from build123d import *

# Parameters (mm, degrees)
BOX078_W               = 3
BOX078_H               = 15
BOX078_DEPTH           = 6
BOX042_W               = 3
BOX042_H               = 9
BOX042_DEPTH           = 3
BOX041_W               = 3
BOX041_H               = 15
BOX041_DEPTH           = 6
BOX044_W               = 3
BOX044_H               = 9
BOX044_DEPTH           = 3
BOX043_W               = 3
BOX043_H               = 15
BOX043_DEPTH           = 6
CUT014_PLACEMENT_ANGLE = 180
BOX040_W               = 3
BOX040_H               = 30
BOX040_DEPTH           = 15
BOX079_W               = 3
BOX079_H               = 15
BOX079_DEPTH           = 6


with BuildPart() as cube002:
    # Box078 → Box078 (new body)
    with BuildSketch(Plane(origin=(-3, 60, 15), x_dir=(1, 0, 0), z_dir=(0, 0, 1))):
        with Locations((1.5, 7.5)):
            Rectangle(BOX078_W, BOX078_H)
    extrude(amount=BOX078_DEPTH)


with BuildPart() as obj1:
    # Box042 → Box042 (new body)
    with BuildSketch(Plane(origin=(0, 3, 0), x_dir=(1, 0, 0), z_dir=(0, 0, 1))):
        with Locations((1.5, 4.5)):
            Rectangle(BOX042_W, BOX042_H)
    extrude(amount=BOX042_DEPTH)


with BuildPart() as loop004:
    # Box041 → Box041 (new body)
    with BuildSketch(Plane.XY):
        with Locations((1.5, 7.5)):
            Rectangle(BOX041_W, BOX041_H)
    extrude(amount=BOX041_DEPTH)

    # Cut013: cut obj1
    add(obj1.part, mode=Mode.SUBTRACT)


with BuildPart() as loop004_1:
    # Cut013 placement: moved
    add(loop004.part.moved(Location((30, 75, 15))))


with BuildPart() as obj2:
    # Box044 → Box044 (new body)
    with BuildSketch(Plane(origin=(0, 3, 0), x_dir=(1, 0, 0), z_dir=(0, 0, 1))):
        with Locations((1.5, 4.5)):
            Rectangle(BOX044_W, BOX044_H)
    extrude(amount=BOX044_DEPTH)


with BuildPart() as loop005:
    # Box043 → Box043 (new body)
    with BuildSketch(Plane.XY):
        with Locations((1.5, 7.5)):
            Rectangle(BOX043_W, BOX043_H)
    extrude(amount=BOX043_DEPTH)

    # Cut014: cut obj2
    add(obj2.part, mode=Mode.SUBTRACT)


with BuildPart() as loop005_1:
    # Cut014 placement: moved
    add(loop005.part.moved(Location((33, 75, 0))).rotate(Axis((33, 75, 0), (0, 1, 0)), CUT014_PLACEMENT_ANGLE))


with BuildPart() as sideplate002:
    # Box040 → Box040 (new body)
    with BuildSketch(Plane(origin=(30, 60, 0), x_dir=(1, 0, 0), z_dir=(0, 0, 1))):
        with Locations((1.5, 15)):
            Rectangle(BOX040_W, BOX040_H)
    extrude(amount=BOX040_DEPTH)

    # Fusion010: union Loop004, Loop005
    add(loop004_1.part)
    add(loop005_1.part)


with BuildPart() as sideplate002_1:
    # Fusion010 placement: moved
    add(sideplate002.part.moved(Location((-33, 0, 0))))


with BuildPart() as fusion023:
    # Box079 → Box079 (new body)
    with BuildSketch(Plane(origin=(-3, 60, -6), x_dir=(1, 0, 0), z_dir=(0, 0, 1))):
        with Locations((1.5, 7.5)):
            Rectangle(BOX079_W, BOX079_H)
    extrude(amount=BOX079_DEPTH)

    # Fusion023: union Cube002, SidePlate002
    add(cube002.part)
    add(sideplate002_1.part)


solid = fusion023.part
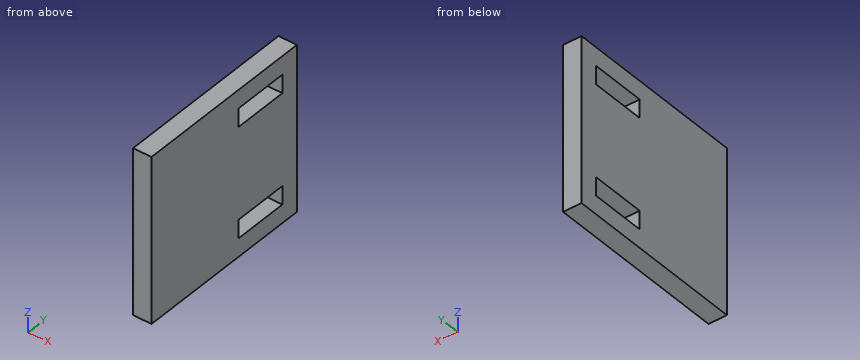
Build history of the part. All positions in model axes, mm. Round coordinates to 2 decimals unless told otherwise and drop trailing zeros. Loops run counter-clockwise (first coordinate to the right, second up) from the corner with the lowest first, then second, coordinate; pieces in that order, holes last. Notation, with made-up numbers: (-23, 30) -> (13, 30) arc R24 cw to (13, 53) -> close; hole circle Ø7 at (61, 37.25). An arc over 180 degrees is marked (long way). One line per item, written item: value. Start each with the question number.
Q1. Probe line 1 along Z through (x, y) = (-1.3, 82.75); line 2 along Y through (x, z) = (-2.25, -2.5). List the from-to ranges inside material, lowest first.
Q2. Cut at C-C on z = 16. List the corners of the cut face in (x, y), plus the area to 3 significant figures.
Q3. Cut at A-A on y = 86.25. List the corners of the cut face in (x, z).
Q4. Cut at B-B on x = -1.5. List the corners of the cut face in (y, z), plus the area to 3 significant figures.
Computed:
1. line 1: -6 to -3, 0 to 15, 18 to 21
1. line 2: 60 to 78, 87 to 90
2. outline: (-3, 60) -> (0, 60) -> (0, 78) -> (-3, 78) -> close; (-3, 87) -> (0, 87) -> (0, 90) -> (-3, 90) -> close
2. area: 63.0 mm²
3. outline: (-3, -6) -> (0, -6) -> (0, -3) -> (-3, -3) -> close; (-3, 0) -> (0, 0) -> (0, 15) -> (-3, 15) -> close; (-3, 18) -> (0, 18) -> (0, 21) -> (-3, 21) -> close
4. outline: (60, -6) -> (90, -6) -> (90, 21) -> (60, 21) -> close; hole (78, -3) -> (87, -3) -> (87, 0) -> (78, 0) -> close; hole (78, 15) -> (87, 15) -> (87, 18) -> (78, 18) -> close
4. area: 756 mm²
